```python
from build123d import *

# Parameters (mm, degrees)
BOSS_EXTRUDE1_DEPTH      = 1.5
BOSS_EXTRUDE1_DEPTH_BACK = 1.5
BODY_MOVE_COPY1_ANGLE    = 90


with BuildPart() as part:
    # Sketch2 → Boss-Extrude1 (new, two sides: drawn at the far end of the back side and taken through both)
    with BuildSketch(Plane(origin=(0, 0, 0), x_dir=(1, 0, 0), z_dir=(0, 1, 0)).offset(-BOSS_EXTRUDE1_DEPTH_BACK)):
        with BuildLine():
            Line((1.6, 1.425), (0, 1.425))
            Line((0, 1.425), (0, 7))
            ThreePointArc((0, 7), (0.805347718, 6.953518178), (1.6, 6.814690015))
            ThreePointArc((1.6, 6.814690015), (7, 0), (1.6, -6.814690015))
            Line((1.6, -6.814690015), (1.6, -1.425))
            Line((1.6, -1.425), (4.5, -1.425))
            Line((4.5, -1.425), (4.5, 1.425))
            Line((4.5, 1.425), (1.6, 1.425))
        make_face()
    extrude(amount=BOSS_EXTRUDE1_DEPTH + BOSS_EXTRUDE1_DEPTH_BACK)


with BuildPart() as part_1:
    # Body-Move/Copy1: moved
    add(part.part.rotate(Axis((0, 0, 0), (0, 0, 1)), BODY_MOVE_COPY1_ANGLE))


solid = part_1.part
```
Input: part model. Units: mm. Frame: model coordinates. A direction names the side the tool comes from. Round coordinates to 2 decimals unless told otherwise and drop trailing zeros. Loops run counter-clockwise (first coordinate to the right, second up) from the corner with the lowest first, then second, coordinate; pieces in that order, holes last. Notation, with made-up numbers: (74.5, 52.5) -> (109.5, 52.5) arc R8 ccw to (109.5, 63.5) -> close; hole circle Ø7 at (28, 38). An arc over 180 degrees is marked (long way). Use one line per item in the form item = value. Start each with the question number.
Item 1: Mould query, pull axis Z, two halves, no side actions, for faces 1 (the face through (0, 3, 1.425)), 2 (the face through (0, 4.5, 0)), 3 (the face through (-1.5, 4, -2)). Classes: pulls with the +Z half, pulls with the -Z half, needs draft (parallel to the pull), parting line crosses it, or undercut.
Item 2: Section query A-A on y = 2.75. Return the cut outline in (x, z) (3 decimals), then the cut area to 3 significant figures.
Item 3: Contact query for a flat-ended pin moving along its axis: pin 1 Ø1.5 at (x, y) = (-0.5, 2.5) entering from -Z. Output: stop coordinate, or through.
Item 4: Material intervals for L1, parallel to Z at x = -0.1, y = 2.75 (3 decimals); L2, parallel to Z at x = -0.5, y = 2 (3 decimals); L3, parallel to Y at x = -1.1, z = 2.5, sorted ascending. Write a range as from..to.
Item 5: Section query C-C on z = -5.25. Return the cut outline in (x, y), then the cut area to 3 significant figures.
Item 6: Section query D-D on y = 1. Return the cut outline in (x, z) (3 decimals).
Item 7: Section query B-B on x = 1.2. Return the cut outline in (y, z) (3 decimals).
Item 8: Set-up query: faces 4 (the face through (0, 2, -1.425)), 5 (the face through (0, 0, -4)), 6 (the face through (0, 1.6, 4)). Return all of +Z, -Z, +X, -X, +Y, -Y with unobstructed straight access to the full face (end or side cutting, diameter ignored); none if empty.
Ans:
q1.face_1 = undercut
q1.face_2 = undercut
q1.face_3 = needs draft
q2.outline = (-1.5, -6.437) -> (1.5, -6.437) -> (1.5, -1.425) -> (-1.5, -1.425) -> close; (-1.5, 1.425) -> (1.5, 1.425) -> (1.5, 6.437) -> (-1.5, 6.437) -> close
q2.area = 30.1 mm^2
q3.pin_1 = -6.78
q4.L1 = -6.437..-1.425, 1.425..6.437
q4.L2 = -6.708..-1.425, 1.425..6.708
q4.L3 = 1.6..6.54
q5.outline = (-1.5, 0) -> (1.5, 0) -> (1.5, 4.63) -> (-1.5, 4.63) -> close
q5.area = 13.9 mm^2
q6.outline = (-1.5, -6.928) -> (1.5, -6.928) -> (1.5, -1.425) -> (-1.5, -1.425) -> close
q7.outline = (0, -7) arc R7 ccw to (1.6, 6.815) -> (1.6, 1.425) -> (4.5, 1.425) -> (4.5, -1.425) -> (0, -1.425) -> close
q8.face_4 = +X, -X, -Y
q8.face_5 = +Z, -Z, +X, -X, -Y
q8.face_6 = +Z, +X, -X, -Y
